Input: dimensioned drawing with shaded views. Units: mm. Origin: part minimum x, y, z. Coordinates: 2 decimals unless noted, no trailing zeros. Loops run counter-clockwise (first coordinate to the right, second up) from the corner with the lowest first, then second, coordinate; pieces in that order, holes last. Notation, with made-up numbers: M -17,38 L -9,38 A22 cw -9,64 Z; hole C -19,51.5 d9. An arc over 180 degrees is marked long. Write item = value, one per line. Start each with the question number.
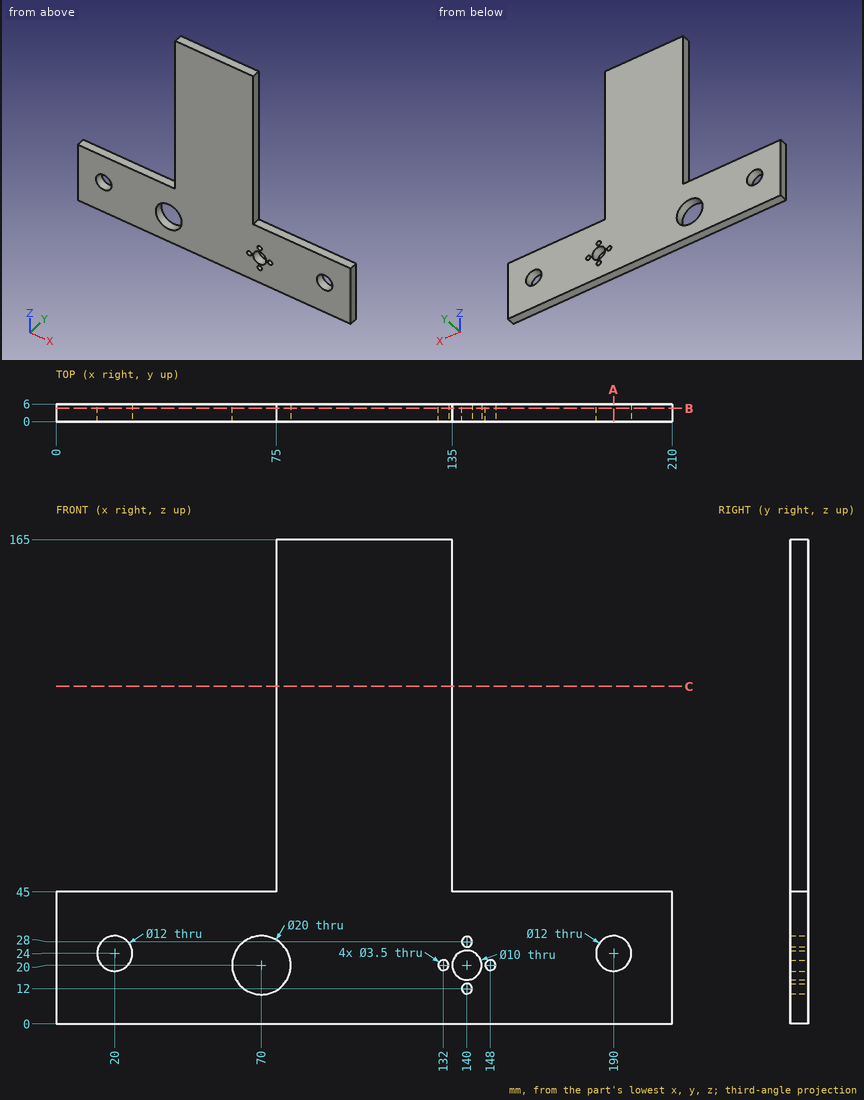
Item 1: Section query A-A (x = 190). Return the cut outline in (y, z).
Item 2: Line query: line 1 (Z direction, x = 140, y = 2.95); line 2 (Z direction, x = 70, y = 3.15); line 3 (Z direction, x = 20, y = 4.55). Output: solid intervals per line, ascending. Write a range as from..to.
Item 3: Section query B-B (y = 4.55). Count the separate pieces of the cut face and the enclosed holes in it, plus the area to 3 significant figures.
Item 4: Section query C-C (z = 115). Return the cut outline in (x, y), plus the area to 3 significant figures.
Item 5: First-contact query: pin 1 (1.8 mm diameter, centred on y = 2, z = 88.5, fed in from +X); pin 2 (1.8 mm diameter, centred on y = 2.5, z = 86, fed in from -X). Flat tips, straight axial feed; report the tip coordinate or a pass-through.
Verdict:
q1.outline = M 0,0 L 6,0 L 6,18 L 0,18 Z; M 0,30 L 6,30 L 6,45 L 0,45 Z
q2.line_1 = 0..10.25, 13.75..15, 25..26.25, 29.75..45
q2.line_2 = 0..10, 30..45
q2.line_3 = 0..18, 30..45
q3.separate_pieces = 1
q3.enclosed_holes = 8
q3.area = 16,000 mm2
q4.outline = M 75,0 L 135,0 L 135,6 L 75,6 Z
q4.area = 360 mm2
q5.pin_1 = 135
q5.pin_2 = 75
